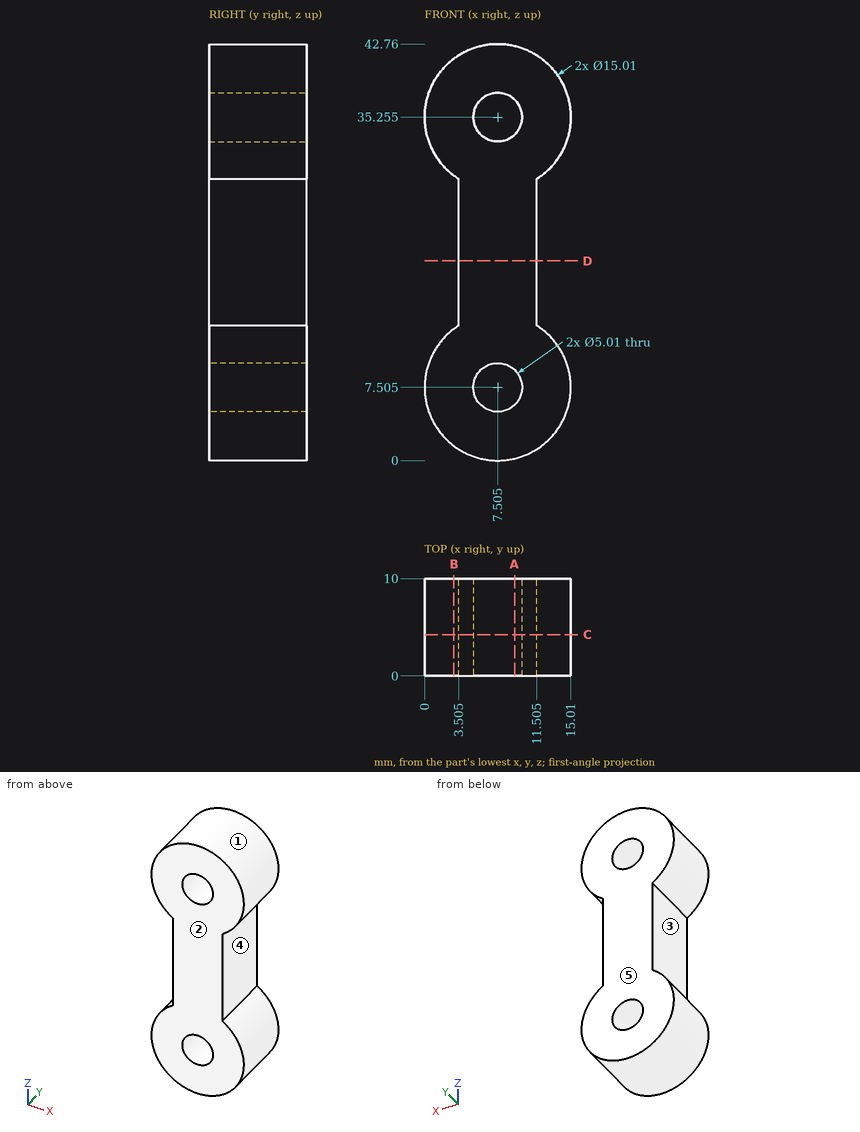
For this review, use the dimensioned drawing (mm, ordinates from the lowest corner) and the shaded views. A direction names the side the tool comes from. Give positions to 0.01 mm unless a question says otherwise; leave off trailing zeros. Order: outer loops, then holes, each group sorted by start corner. A loop starts at its lowest first (then second) coordinate and runs counter-clockwise, first axis right, second up.
1) Take a section at A-A (x = 9.25). Give the boundary of the cut face in (y, z), then the cut area to 3 significant figures.
2) Take a section at B-B (x = 3). Give the boundary of the cut face in (y, z).
3) Insertion check: pin 1 (3 mm diameter, centred on y = 4, z = 24, fed in from +X) (3 decimals); pin 2 (3 mm diameter, centred on y = 4, z = 34.5, fed in from +X); pin 3 (5 mm diameter, centred on y = 3, z = 20.5, fed in from -X) (3 decimals); pin 4 (5 mm diameter, centred on y = 2.5, z = 28, fed in from -X). Each pin has a flat end and moves straight along its axis. Give the tip position at first contact, or say it passes through.
4) For the marked faces 3, 4 and 5, list the 3-axis set-ups (+Z, -Z, +X, -X, +Y, -Y) from which the entire face can be reached by the end or side of a thin tool; tool diameter is ignored.
5) Wall thickness on line 1 (X direction, y = 4.5, z = 7.5); line 2 (Z direction, x = 6, y = 4.75); line 3 (X direction, y = 6.75, z = 25) (3 decimals): over which ranges is each line inside the solid? List them lowest first.
6) The part is to be moulded in two halves that separate along Z. For the marked faces 1 and 2, say which applies: released by +Z, released by -Z, zero draft, split by the parting line, or undercut.
7) Take a section at D-D (z = 20.5). Give the boundary of the cut face in (x, y) (3 decimals).
8) Take a section at C-C (y = 4.25). Give the boundary of the cut face in (x, z) (3 decimals).
Derived:
1. outline: (0, 0.21) - (10, 0.21) - (10, 5.71) - (0, 5.71) - close; (0, 9.3) - (10, 9.3) - (10, 33.46) - (0, 33.46) - close; (0, 37.05) - (10, 37.05) - (10, 42.55) - (0, 42.55) - close
1. area: 352 mm2
2. outline: (0, 1.5) - (10, 1.5) - (10, 13.51) - (0, 13.51) - close; (0, 29.25) - (10, 29.25) - (10, 41.26) - (0, 41.26) - close
3. pin 1: stops at x = 11.505
3. pin 2: stops at x = 15.01
3. pin 3: stops at x = 3.505
3. pin 4: stops at x = 1.7
4. face 3: -X, +Y, -Y
4. face 4: +X, +Y, -Y
4. face 5: +Z, -Z, +X, -X, +Y
5. line 1: x = 0 to 5, 10.01 to 15.01
5. line 2: z = 0.15 to 5.5, 9.51 to 33.25, 37.26 to 42.61
5. line 3: x = 3.505 to 11.505
6. face 1: undercut
6. face 2: zero draft
7. outline: (3.505, 0) - (11.505, 0) - (11.505, 10) - (3.505, 10) - close
8. outline: (3.505, 13.855) arc R7.505 ccw (long way) to (11.505, 13.855) - (11.505, 28.905) arc R7.505 ccw (long way) to (3.505, 28.905) - close; hole circle Ø5.01 at (7.505, 7.505); hole circle Ø5.01 at (7.505, 35.255)
